```python
from build123d import *

# Parameters (mm, degrees)
SKETCH1_W           = 50.565864073
SKETCH1_H           = 126.812282012
BOSS_EXTRUDE2_DEPTH = 38.354
SHELL1_T            = 2.54
SKETCH5_W           = 7.375102077
SKETCH5_H           = 11.361908509
SKETCH5_W_2         = 7.375102076
CUT_EXTRUDE3_DEPTH  = 1.27
SKETCH8_W           = 35.70829539
SKETCH8_H           = 19.028689215
CUT_EXTRUDE4_DEPTH  = 1.27


with BuildPart() as part:
    # Sketch1 → Boss-Extrude2 (new body)
    with BuildSketch(Plane.XY):
        with Locations((25.282932037, -63.406141006)):
            Rectangle(SKETCH1_W, SKETCH1_H)
    extrude(amount=BOSS_EXTRUDE2_DEPTH)

    # Shell1 (no face opened: a closed hollow body)
    add(offset(amount=-SHELL1_T, mode=Mode.PRIVATE), mode=Mode.SUBTRACT)

    # Sketch5 → Cut-Extrude3 (cut)
    with BuildSketch(Plane.XY.offset(38.354)):
        with Locations((32.253317714, -115.98095696)):
            Rectangle(SKETCH5_W, SKETCH5_H)
        with Locations((15.859200433, -116.102649257)):
            Rectangle(SKETCH5_W_2, SKETCH5_H)
        with Locations((32.124042774, -7.70128789)):
            Rectangle(SKETCH5_W, SKETCH5_H)
        with Locations((15.729925493, -7.822980187)):
            Rectangle(SKETCH5_W_2, SKETCH5_H)
    extrude(amount=-CUT_EXTRUDE3_DEPTH, mode=Mode.SUBTRACT)

    # Sketch8 → Cut-Extrude4 (cut)
    with BuildSketch(Plane(origin=(0, 0, 0), x_dir=(-1, 0, 0), z_dir=(0, 0, -1))):
        with Locations((-25.453839923, -109.412856846)):
            Rectangle(SKETCH8_W, SKETCH8_H)
    extrude(amount=-CUT_EXTRUDE4_DEPTH, mode=Mode.SUBTRACT)


solid = part.part
```
Check sheet for the modelled part. Datum: model origin and axes. Units: mm. A direction names the side the tool comes from. Coordinates: 2 decimals unless noted, no trailing zeros. Write each loop counter-clockwise with the first axis right and the second up, starting at its lowest first coordinate (ties: lowest second). Pieces come first, ordered by that corner, then holes. Notation, with made-up numbers: M 13.25,-27.75 L 43.25,-27.75 A21 cw 43.25,-7.75 Z; hole C 2,-13.75 d10. An arc over 180 degrees is marked long. Write item = value, one per line. Start each with the question number.
1. Sectioned sample at B-B (x = 40). Record the cut outline in (y, z), then the cut area to 3 significant figures.
2. Sectioned sample at C-C (z = 28.5). Record the cut outline in (x, y).
3. Mould release check, pull along X, two halves, no side actions. Record for faces 1 (the flat face through (16, -116, 37.084)), 2 (the flat face through (25, 0, 19)), 3 (the flat face through (0, -64, 19)): pulls with the +X half, pulls with the -X half, needs draft (parallel to the pull), parting line crosses it, or undercut.
4. Sectioned sample at A-A (y = -30.5). Record the cut outline in (x, z), then the cut area to 3 significant figures.
5. Tool access check on faces 4 (the flat face through (26, -109, 1.27)), 5 (the flat face through (16, -8, 37.084)), 6 (the flat face through (25, -124.272, 19)). Record the directions out of +Z, -Z, +X, -X, +Y, -Y that give a thin tool (end or side, any length) a straight path to the whole face; none if there is none.
6. Go/stop test with a flat-tipped pin: pin 1 (3.5 mm diameter, centred on x = 14, y = -6, fed in from +Z). Record where the tip stops, or that it passes through.
7. Thickness scan on probe 1 along Y at (x, z) = (47.5, 7.5); probe 2 along X at (y, z) = (-30.5, 6.5); probe 3 along Z at (x, y) = (16.5, -101.5). Record the ranges inside material, lowest first.
8. Sectioned sample at D-D (x = 34). Record the cut outline in (y, z).
The answers:
q1.outline = M -126.81,0 L -118.93,0 L -118.93,1.27 L -99.9,1.27 L -99.9,0 L 0,0 L 0,38.35 L -126.81,38.35 Z; hole M -124.27,2.54 L -2.54,2.54 L -2.54,35.81 L -124.27,35.81 Z
q1.area = 789 mm²
q2.outline = M 0,-126.81 L 50.57,-126.81 L 50.57,0 L 0,0 Z; hole M 2.54,-124.27 L 48.03,-124.27 L 48.03,-2.54 L 2.54,-2.54 Z
q3.face_1 = undercut
q3.face_2 = needs draft
q3.face_3 = pulls with the -X half
q4.outline = M 0,0 L 50.57,0 L 50.57,38.35 L 0,38.35 Z; hole M 2.54,2.54 L 48.03,2.54 L 48.03,35.81 L 2.54,35.81 Z
q4.area = 426 mm²
q5.face_4 = -Z
q5.face_5 = +Z
q5.face_6 = none
q6.pin_1 = 37.08
q7.probe_1 = -126.81 to -124.27, -2.54 to 0
q7.probe_2 = 0 to 2.54, 48.03 to 50.57
q7.probe_3 = 1.27 to 2.54, 35.81 to 38.35
q8.outline = M -126.81,0 L -118.93,0 L -118.93,1.27 L -99.9,1.27 L -99.9,0 L 0,0 L 0,38.35 L -2.02,38.35 L -2.02,37.08 L -13.38,37.08 L -13.38,38.35 L -110.3,38.35 L -110.3,37.08 L -121.66,37.08 L -121.66,38.35 L -126.81,38.35 Z; hole M -124.27,2.54 L -2.54,2.54 L -2.54,35.81 L -124.27,35.81 Z
